from build123d import *

# Parameters (mm, degrees)
EXTRUDE_1_DEPTH     = 6
SKETCH_2_R          = 1.55
CUT_EXTRUDE_1_DEPTH = 6
FILLET_2_R          = 3
SKETCH_3_W          = 2
SKETCH_3_H          = 0.85
CUT_EXTRUDE_2_DEPTH = 5.5
SKETCH_4_W          = 1.15
SKETCH_4_H          = 0.85
SKETCH_4_W_2        = 2


with BuildPart() as part:
    # 草图1 → 凸台-拉伸1 (new body)
    with BuildSketch(Plane.XY):
        with BuildLine():
            Line((-5.5, 14), (-5.5, 5.75))
            Line((-5.5, 5.75), (0, 5.75))
            ThreePointArc((0, 5.75), (5.75, 0), (0, -5.75))
            Line((0, -5.75), (-5.5, -5.75))
            Line((-5.5, -5.75), (-5.5, -14))
            Line((-5.5, -14), (-2.5, -14))
            Line((-2.5, -14), (-2.5, -8.25))
            Line((-2.5, -8.25), (0, -8.25))
            ThreePointArc((0, -8.25), (8.25, 0), (0, 8.25))
            Line((0, 8.25), (-2.5, 8.25))
            Line((-2.5, 8.25), (-2.5, 14))
            Line((-2.5, 14), (-5.5, 14))
        make_face()
    extrude(amount=EXTRUDE_1_DEPTH)

    # 草图2 → 切除-拉伸1 (cut)
    with BuildSketch(Plane(origin=(-2.5, 0, 0), x_dir=(0, 0, -1), z_dir=(1, 0, 0))):
        with Locations(Location((-3, -11, 0), (0, 0, 90))):
            Circle(SKETCH_2_R)
        with Locations(Location((-3, 11, 0), (0, 0, 90))):
            Circle(SKETCH_2_R)
    extrude(amount=-CUT_EXTRUDE_1_DEPTH, mode=Mode.SUBTRACT)

    # 圆角2
    fillet_2_edges = [part.edges().sort_by_distance(p)[0] for p in [
        (-4, -14, 0),
        (-4, -14, 6),
        (-4, 14, 0),
        (-4, 14, 6),
    ]]
    fillet(fillet_2_edges, radius=FILLET_2_R - 0.0001)  # a hair under: the kernel refuses the full size

    # 草图3 → 切除-拉伸2 (cut)
    with BuildSketch(Plane.ZY.offset(5.5)):
        with Locations((0.15, 6.175)):
            Rectangle(SKETCH_3_W, SKETCH_3_H)
        with Locations((3, 6.175)):
            Rectangle(SKETCH_3_W, SKETCH_3_H)
        with Locations((5.85, -6.175)):
            Rectangle(SKETCH_3_W, SKETCH_3_H)
        with Locations((5.85, 6.175)):
            Rectangle(SKETCH_3_W, SKETCH_3_H)
        with Locations((3, -6.175)):
            Rectangle(SKETCH_3_W, SKETCH_3_H)
        with Locations((0.15, -6.175)):
            Rectangle(SKETCH_3_W, SKETCH_3_H)
    extrude(amount=-CUT_EXTRUDE_2_DEPTH, mode=Mode.SUBTRACT)

    # 草图4 → 切除-旋转1 (revolve, cut)
    with BuildSketch(Plane.ZY):
        with Locations((5.425, 6.175)):
            Rectangle(SKETCH_4_W, SKETCH_4_H)
        with Locations((3, 6.175)):
            Rectangle(SKETCH_4_W_2, SKETCH_4_H)
        with Locations((0.575, 6.175)):
            Rectangle(SKETCH_4_W, SKETCH_4_H)
    revolve(axis=Axis((0, 0, 0), (0, 0, 1)), mode=Mode.SUBTRACT)


solid = part.part
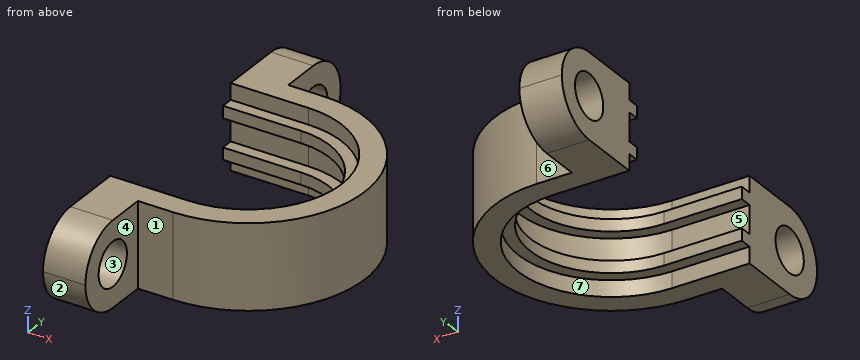
Read the model definition and answer for the solid it produces. Units are mm, in the model's axes. Face numbers are marked on the shaded views. A direction names the side the tool comes from. Round coordinates to 2 decimals unless told otherwise and drop trailing zeros. Write each loop counter-clockwise with the first axis right and the second up, starting at its lowest first coordinate (ties: lowest second). Pieces come first, ordered by that corner, then holes.
Q1. Find section D-D on y = 0. Determine the outline of the cut face in (x, z).
Values:
outline: (5.75, 1.15) - (6.6, 1.15) - (6.6, 0) - (8.25, 0) - (8.25, 6) - (6.6, 6) - (6.6, 4.85) - (5.75, 4.85) - (5.75, 4) - (6.6, 4) - (6.6, 2) - (5.75, 2) - close
Q2. Find section A-A on x = 2.25. Determine the outline of the cut face in (y, z).
Values:
outline: (-7.94, 0) - (-6.2, 0) - (-6.2, 1.15) - (-5.29, 1.15) - (-5.29, 2) - (-6.2, 2) - (-6.2, 4) - (-5.29, 4) - (-5.29, 4.85) - (-6.2, 4.85) - (-6.2, 6) - (-7.94, 6) - close; (5.29, 1.15) - (6.2, 1.15) - (6.2, 0) - (7.94, 0) - (7.94, 6) - (6.2, 6) - (6.2, 4.85) - (5.29, 4.85) - (5.29, 4) - (6.2, 4) - (6.2, 2) - (5.29, 2) - close
Q3. Find section C-C on y = 12. Determine the outline of the cut face in (x, z), and give its area (3 significant figures).
Values:
outline: (-5.5, 0.17) - (-2.5, 0.17) - (-2.5, 1.82) - (-5.5, 1.82) - close; (-5.5, 4.18) - (-2.5, 4.18) - (-2.5, 5.83) - (-5.5, 5.83) - close
area: 9.87 mm2
Q4. Straight lines are drawn through the part: line 1 (Z direction, x = -3.4, y = -11); line 2 (Y direction, x = -1, z = 4.3); line 3 (Y direction, x = -2.25, z = 2.45). For each, find the intervals that lie inside material, in ascending order.
Values:
line 1: z = 0 to 1.45, 4.55 to 6
line 2: y = -8.25 to -5.75, 5.75 to 8.25
line 3: y = -8.25 to -6.6, 6.6 to 8.25
Q5. Flat-ended cylindrical pins translate along their axes: P1, Ø3.5, axis at x = 1.5, y = 2.5, coming from the -Z side; P2, Ø4, axis at x = 4.5, y = 0, coming from the +Z side; P3, Ø0.8, axis at x = -0.5, z = 2, coming from the -Y side; P4, Ø6, axis at x = 4.5, y = -4.5, coming from the +Z side. Find the tip coordinate at first contact, or state that the pin passes through.
Values:
P1: passes through
P2: stops at z = 4.85
P3: stops at y = -8.25
P4: stops at z = 6
Q6. The mould has two halves that part along Z. Classify the marked faces 1, 2 and 3: released by +Z, released by -Z, zero draft, split by the parting line, or undercut.
Values:
face 1: zero draft
face 2: released by -Z
face 3: undercut
Q7. A tool of negligible diameter and unlimited length cuts with its end or side. For the marked faces 4, 5, 6 and 7, from which of +Z, -Z, +X, -X, +Y, -Y can it reach the whole face along a straight path? Write none if from no direction.
Values:
face 4: +Z, -Z, +X, -Y
face 5: -X
face 6: +Z, -Z, +X, +Y
face 7: -Z, -X
Q8. Find section B-B on z = 3.6. Determine the outline of the cut face in (x, y).
Values:
outline: (-5.5, -13.94) - (-2.5, -13.94) - (-2.5, -12.43) - (-5.5, -12.43) - close; (-5.5, -9.57) - (-2.5, -9.57) - (-2.5, -8.25) - (0, -8.25) arc R8.25 ccw to (0, 8.25) - (-2.5, 8.25) - (-2.5, 9.57) - (-5.5, 9.57) - (-5.5, 6.6) - (0, 6.6) arc R6.6 cw to (0, -6.6) - (-5.5, -6.6) - close; (-5.5, 12.43) - (-2.5, 12.43) - (-2.5, 13.94) - (-5.5, 13.94) - close
